from build123d import *

# Parameters (mm, degrees)
F0_W     = 12.7
F0_H     = 63.5
F1_DEPTH = 63.5
F2_W     = 63.5
F2_H     = 12.7
F3_DEPTH = 47.624812


with BuildPart() as f1:
    # F0 (on Front) → F1 (new body)
    with BuildSketch(Plane.XZ):
        with Locations((6.35, -31.75)):
            Rectangle(F0_W, F0_H)
    extrude(amount=F1_DEPTH)

    # F0 (on Front) + F2 (on Front) → F3 (join)
    with BuildSketch(Plane.XZ):
        with Locations((6.35, -31.75)):
            Rectangle(F0_W, F0_H)
    with BuildSketch(Plane.XZ):
        with Locations((31.75, -6.35)):
            Rectangle(F2_W, F2_H)
    extrude(amount=F3_DEPTH)


solid = f1.part
The listing builds one solid part. Answer for the finished solid, in the listing's coordinates (mm). A direction names the side the tool comes from. Coordinates: 2 decimals unless noted, no trailing zeros. Loops run counter-clockwise (first coordinate to the right, second up) from the corner with the lowest first, then second, coordinate; pieces in that order, holes last. Notation, with made-up numbers: (-29.75, 60.5) -> (21.25, 60.5) arc R16 cw to (21.25, 64.5) -> close; hole circle Ø10 at (-26, 70). An arc over 180 degrees is marked (long way). Answer in a Markdown table with one row per item. Add a question column.
1. Flat-ended cylindrical pins translate along their axes: P1, Ø14.5, axis at x = 48, y = -34.5, coming from the -Z side; P2, Ø8, axis at y = -52, z = -35, coming from the +X side; P3, Ø8, axis at x = 13.5, z = -16, coming from the +Y side; P4, Ø10, axis at x = 48, z = -6, coming from the -Y side. Find the tip coordinate at first contact, or state that the pin passes through.
2. For faces 1 (the flat face through (38, -23, -12.7)), 2 (the flat face through (6, -31, -63.5)), 3 (the flat face through (38, -47.625, -6)), determine the directions among +Z, -Z, +X, -X, +Y, -Y from which every point of the face is accessible in a straight line to the end or side of a thin tool.
3. The part is cut by section C-C, the plane z = -58.5. Write down the section's boundary in (x, y).
4. The part is cut by section A-A, the plane y = -25. Write down the section's boundary in (x, z), then the cut area to 3 significant figures.
5. Consider line 1 (Z direction, x = 27, y = -22.5); line 2 (X direction, y = -23, z = -53.5); line 3 (Y direction, x = 56.5, z = -6). Determine where each line is inside the solid, lowest interval first. Write a range as [from, to].
6. The part is cut by section B-B, the plane x = 47. Write down the section's boundary in (y, z), then the cut area to 3 significant figures.
Answer below:
| question | item | result |
|---|---|---|
| 1 | P1 | z = -12.7 |
| 1 | P2 | x = 12.7 |
| 1 | P3 | y = 0 |
| 1 | P4 | y = -47.62 |
| 2 | face 1 | -Z, +X, +Y, -Y |
| 2 | face 2 | -Z, +X, -X, +Y, -Y |
| 2 | face 3 | +Z, -Z, +X, -Y |
| 3 | outline | (0, -63.5) -> (12.7, -63.5) -> (12.7, 0) -> (0, 0) -> close |
| 4 | outline | (0, -63.5) -> (12.7, -63.5) -> (12.7, -12.7) -> (63.5, -12.7) -> (63.5, 0) -> (0, 0) -> close |
| 4 | area | 1,450 mm2 |
| 5 | line 1 | [-12.7, 0] |
| 5 | line 2 | [0, 12.7] |
| 5 | line 3 | [-47.62, 0] |
| 6 | outline | (-47.62, -12.7) -> (0, -12.7) -> (0, 0) -> (-47.62, 0) -> close |
| 6 | area | 605 mm2 |
